The model under review builds one solid part; all positions refer to its coordinate system, in mm. A direction names the side the tool comes from. Give positions to 0.01 mm unless a question says otherwise; leave off trailing zeros. Loops run counter-clockwise (first coordinate to the right, second up) from the corner with the lowest first, then second, coordinate; pieces in that order, holes last. Notation, with made-up numbers: M -10.75,60.25 L 38.25,60.25 A23 ccw 38.25,86.25 Z; hole C -3,36 d8. An arc over 180 degrees is marked long. Return JSON: item names as keys, results as strings.
```python
from build123d import *

# Parameters (mm, degrees)
F0_W      = 60
F0_H      = 47
F1_DEPTH  = 16
F2_W      = 58
F2_H      = 45
F3_DEPTH  = 0.8
F4_W      = 56
F4_H      = 43
F5_DEPTH  = 0.5
F7_DEPTH  = 60
F9_DEPTH  = 60.001
F11_DEPTH = 60.001
F14_W     = 15.5
F14_H     = 9
F15_DEPTH = 25
F9_FACE_W = 60
F9_FACE_H = 16.2788205961
F17_DEPTH = 1.5


with BuildPart() as f1:
    # F0 (on Top) → F1 (new body)
    with BuildSketch(Plane.XY):
        Rectangle(F0_W, F0_H)
    extrude(amount=F1_DEPTH)

    # F2 (on face) → F3 (join)
    with BuildSketch(Plane(origin=(0, 0, 0), x_dir=(1, 0, 0), z_dir=(0, 0, -1))):
        Rectangle(F2_W, F2_H)
    extrude(amount=F3_DEPTH)

    # F4 (on face) → F5 (cut)
    with BuildSketch(Plane(origin=(0, 0, -0.8), x_dir=(1, 0, 0), z_dir=(0, 0, -1))):
        Rectangle(F4_W, F4_H)
    extrude(amount=-F5_DEPTH, mode=Mode.SUBTRACT)

    # F6 (on face) → F7 (join)
    with BuildSketch(Plane.YZ.offset(30)):
        Polygon((26.5, 16), (23.5, 16), (23.5, 0), align=None)
    extrude(amount=-F7_DEPTH)

    # F8 (on face) → F9 (cut, through all)
    with BuildSketch(Plane.YZ.offset(30)):
        Polygon((-20.5, 16), (-23.5, 16), (-23.5, 0), align=None)
    extrude(amount=-F9_DEPTH, mode=Mode.SUBTRACT)

    # F10 (on face) → F11 (cut, through all)
    with BuildSketch(Plane.YZ.offset(30)):
        Polygon((-4.261999952, 5.4947938472), (-1, 16), (-18, 16), (-19.0636169243, 10.0950259071), align=None)
    extrude(amount=-F11_DEPTH, mode=Mode.SUBTRACT)

    # F14 (on plane+point) → F15 (cut)
    with BuildSketch(Plane.XZ.offset(-15.5)):
        with Locations((0, 4.5)):
            Rectangle(F14_W, F14_H)
    extrude(amount=-F15_DEPTH, mode=Mode.SUBTRACT)

    # F16 (on face) + F9_face (on face) → F17 (cut)
    with BuildSketch(Plane(origin=(0, 1.1819033976, 3.8028693253), x_dir=(1, 0, 0), z_dir=(0, 0.2967891652, 0.9549430305))):
        with BuildLine():
            ThreePointArc((7.5, -15.4507624286), (9.5, -13.4507624286), (7.5, -11.4507624286))
            Line((7.5, -11.4507624286), (-7.5, -11.4507624286))
            ThreePointArc((-7.5, -11.4507624286), (-9.5, -13.4507624286), (-7.5, -15.4507624286))
            Line((-7.5, -15.4507624286), (7.5, -15.4507624286))
        make_face()
    with BuildSketch(Plane(origin=(0, -22, 8), x_dir=(1, 0, 0), z_dir=(0, -0.9828721869, 0.1842885351))):
        Rectangle(F9_FACE_W, F9_FACE_H)
    extrude(amount=-F17_DEPTH, dir=(0, 0.2967891652, 0.9549430305), mode=Mode.SUBTRACT)


solid = f1.part
```
1) Consider section C-C on x = -1. Write out the cut boundary in (y, z), then the cut area to 3 significant figures.
From the geometry:
{"outline": "M -23.5,0 L -22.5,0 L -22.5,-0.8 L -21.5,-0.8 L -21.5,-0.3 L 21.5,-0.3 L 21.5,-0.8 L 22.5,-0.8 L 22.5,0 L 15.5,0 L 15.5,9 L 25.19,9 L 26.5,16 L -1,16 L -4.26,5.49 L -9.75,7.2 L -10.2,5.77 L -14.02,6.96 L -13.57,8.39 L -19.06,10.1 L -18,16 L -20.5,16 Z", "area": "545 mm²"}
2) The part is to be moulded in two halves that separate along Z. For faces 1 (the face through (0.42, 25.312, 9.666)), 2 (the face through (0, -19, 16)), 3 (the face through (7.75, 20, 4)), say which applies: released by +Z, released by -Z, zero draft, split by the parting line, or undercut.
From the geometry:
{"face 1": "released by -Z", "face 2": "released by +Z", "face 3": "undercut"}
3) Insertion check: pin 1 (10 mm diameter, centred on x = -2, z = 5, fed in from +Y) (3 decimals); pin 2 (1.5 mm diameter, centred on x = -6, z = 1.5, fed in from -Y); pin 3 (0.6 mm diameter, centred on y = 4, z = -0.5, fed in from +X). Each pin has a flat end and moves straight along its axis. Give the tip position at first contact, or say it passes through.
From the geometry:
{"pin 1": "y = 25.375", "pin 2": "y = -23.36", "pin 3": "x = 29"}
4) Consider section B-B on z = 12.5. Write out the cut boundary in (x, y).
From the geometry:
{"outline": "M -30,-21.16 L 30,-21.16 L 30,-18.63 L -30,-18.63 Z; M -30,-2.09 L 30,-2.09 L 30,25.84 L -30,25.84 Z"}
5) Consider section D-D on z = 4. Write out the cut boundary in (x, y), then the cut area to 3 significant figures.
From the geometry:
{"outline": "M -30,-22.75 L 30,-22.75 L 30,24.25 L 7.75,24.25 L 7.75,15.5 L -7.75,15.5 L -7.75,24.25 L -30,24.25 Z", "area": "2,680 mm²"}
6) Tool access review of faces 4 (the face through (9.5, -11.9, 7.1)), 5 (the face through (0.42, -2.654, 10.674)), 6 (the face through (-30, 7, 6)), 7 (the face through (0, 20, 9)), 8 (the face through (0.42, -18.524, 13.089)): name each direction out of +Z, -Z, +X, -X, +Y, -Y from which nothing blocks a thin tool from reaching the whole face with its end or side.
From the geometry:
{"face 4": "none", "face 5": "+Z, +X, -X", "face 6": "+Z, -Z, -X, +Y, -Y", "face 7": "+Y", "face 8": "+X, -X"}
7) Consider section A-A on y = 12. Write out the cut boundary in (x, z), then the cut area to 3 significant figures.
From the geometry:
{"outline": "M -30,0 L -29,0 L -29,-0.8 L -28,-0.8 L -28,-0.3 L 28,-0.3 L 28,-0.8 L 29,-0.8 L 29,0 L 30,0 L 30,16 L -30,16 Z", "area": "978 mm²"}
8) Wall thickness on L1, parallel to Y at x = -25, z = 13.25; L2, parallel to Z at x = -26, y = 1; L3, parallel to Y at x = 23.5, z = 10.5: over which ranges is each line inside the solid? List them lowest first. Write a range as from..to.
From the geometry:
{"L1": "-21.02..-18.5, -1.85..25.98", "L2": "-0.3..16", "L3": "-21.53..-18.99, -2.71..25.47"}
